Work out the finished part from the listing and answer in its coordinate system (mm). Coordinates: 2 decimals unless noted, no trailing zeros.
1. Find the intervals of material crossed by probe 1 along Y at (x, z) = (0.25, 0.2), in increasing order.
2. The part is cut by section A-A, the plane y = -2.75. Count the separate pieces of the cut face and the enclosed holes in it, then the cut area to 3 significant figures.
3. Determine the mould class of faces 1 (the flat face through (-14.286, -3.7, 0.5)), 2 (the flat face through (-17.111, -5.1, 0.5)), 3 (the flat face through (-2.686, -6.3, 0.5)) for opening direction X: +X half, -X half, draft (parallel to the pull), parting line (faces both ways), or undercut.
```python
from build123d import *

# Parameters (mm, degrees)
F1_W     = 20.491264
F1_H     = 6.716872
F1_W_2   = 0.4
F1_H_2   = 2.2
F2_DEPTH = 1


with BuildPart() as f2:
    # F1 (on face) → F2 (new body)
    with BuildSketch(Plane.XY):
        with Locations((-6.865435, -5.054062)):
            Rectangle(F1_W, F1_H)
        with Locations((-16.485979, -6.256568)):
            Rectangle(F1_W_2, F1_H_2, mode=Mode.SUBTRACT)
        with Locations((-15.685979, -6.256568)):
            Rectangle(F1_W_2, F1_H_2, mode=Mode.SUBTRACT)
        with Locations((-14.885979, -6.256568)):
            Rectangle(F1_W_2, F1_H_2, mode=Mode.SUBTRACT)
        with Locations((-14.085979, -6.256568)):
            Rectangle(F1_W_2, F1_H_2, mode=Mode.SUBTRACT)
        with Locations((-13.285979, -6.256568)):
            Rectangle(F1_W_2, F1_H_2, mode=Mode.SUBTRACT)
        with Locations((-12.485979, -6.256568)):
            Rectangle(F1_W_2, F1_H_2, mode=Mode.SUBTRACT)
        with Locations((-11.685979, -6.256568)):
            Rectangle(F1_W_2, F1_H_2, mode=Mode.SUBTRACT)
        with Locations((-10.885979, -6.256568)):
            Rectangle(F1_W_2, F1_H_2, mode=Mode.SUBTRACT)
        with Locations((-10.085979, -6.256568)):
            Rectangle(F1_W_2, F1_H_2, mode=Mode.SUBTRACT)
        with Locations((-9.285979, -6.256568)):
            Rectangle(F1_W_2, F1_H_2, mode=Mode.SUBTRACT)
        with Locations((-8.485979, -6.256568)):
            Rectangle(F1_W_2, F1_H_2, mode=Mode.SUBTRACT)
        with Locations((-7.685979, -6.256568)):
            Rectangle(F1_W_2, F1_H_2, mode=Mode.SUBTRACT)
        with Locations((-6.885979, -6.256568)):
            Rectangle(F1_W_2, F1_H_2, mode=Mode.SUBTRACT)
        with Locations((-16.485979, -3.656568)):
            Rectangle(F1_W_2, F1_H_2, mode=Mode.SUBTRACT)
        with Locations((-15.685979, -3.656568)):
            Rectangle(F1_W_2, F1_H_2, mode=Mode.SUBTRACT)
        with Locations((-14.885979, -3.656568)):
            Rectangle(F1_W_2, F1_H_2, mode=Mode.SUBTRACT)
        with Locations((-14.085979, -3.656568)):
            Rectangle(F1_W_2, F1_H_2, mode=Mode.SUBTRACT)
        with Locations((-13.285979, -3.656568)):
            Rectangle(F1_W_2, F1_H_2, mode=Mode.SUBTRACT)
        with Locations((-12.485979, -3.656568)):
            Rectangle(F1_W_2, F1_H_2, mode=Mode.SUBTRACT)
        with Locations((-11.685979, -3.656568)):
            Rectangle(F1_W_2, F1_H_2, mode=Mode.SUBTRACT)
        with Locations((-10.885979, -3.656568)):
            Rectangle(F1_W_2, F1_H_2, mode=Mode.SUBTRACT)
        with Locations((-10.085979, -3.656568)):
            Rectangle(F1_W_2, F1_H_2, mode=Mode.SUBTRACT)
        with Locations((-9.285979, -3.656568)):
            Rectangle(F1_W_2, F1_H_2, mode=Mode.SUBTRACT)
        with Locations((-8.485979, -3.656568)):
            Rectangle(F1_W_2, F1_H_2, mode=Mode.SUBTRACT)
        with Locations((-7.685979, -3.656568)):
            Rectangle(F1_W_2, F1_H_2, mode=Mode.SUBTRACT)
        with Locations((-6.885979, -3.656568)):
            Rectangle(F1_W_2, F1_H_2, mode=Mode.SUBTRACT)
        with Locations((-6.085979, -6.256568)):
            Rectangle(F1_W_2, F1_H_2, mode=Mode.SUBTRACT)
        with Locations((-5.285979, -6.256568)):
            Rectangle(F1_W_2, F1_H_2, mode=Mode.SUBTRACT)
        with Locations((-4.485979, -6.256568)):
            Rectangle(F1_W_2, F1_H_2, mode=Mode.SUBTRACT)
        with Locations((-3.685979, -6.256568)):
            Rectangle(F1_W_2, F1_H_2, mode=Mode.SUBTRACT)
        with Locations((-2.885979, -6.256568)):
            Rectangle(F1_W_2, F1_H_2, mode=Mode.SUBTRACT)
        with Locations((-2.085979, -6.256568)):
            Rectangle(F1_W_2, F1_H_2, mode=Mode.SUBTRACT)
        with Locations((-1.285979, -6.256568)):
            Rectangle(F1_W_2, F1_H_2, mode=Mode.SUBTRACT)
        with Locations((-0.485979, -6.256568)):
            Rectangle(F1_W_2, F1_H_2, mode=Mode.SUBTRACT)
        with Locations((0.314021, -6.256568)):
            Rectangle(F1_W_2, F1_H_2, mode=Mode.SUBTRACT)
        with Locations((1.114021, -6.256568)):
            Rectangle(F1_W_2, F1_H_2, mode=Mode.SUBTRACT)
        with Locations((1.914021, -6.256568)):
            Rectangle(F1_W_2, F1_H_2, mode=Mode.SUBTRACT)
        with Locations((2.714021, -6.256568)):
            Rectangle(F1_W_2, F1_H_2, mode=Mode.SUBTRACT)
        with Locations((-6.085979, -3.656568)):
            Rectangle(F1_W_2, F1_H_2, mode=Mode.SUBTRACT)
        with Locations((-5.285979, -3.656568)):
            Rectangle(F1_W_2, F1_H_2, mode=Mode.SUBTRACT)
        with Locations((-4.485979, -3.656568)):
            Rectangle(F1_W_2, F1_H_2, mode=Mode.SUBTRACT)
        with Locations((-3.685979, -3.656568)):
            Rectangle(F1_W_2, F1_H_2, mode=Mode.SUBTRACT)
        with Locations((-2.885979, -3.656568)):
            Rectangle(F1_W_2, F1_H_2, mode=Mode.SUBTRACT)
        with Locations((-2.085979, -3.656568)):
            Rectangle(F1_W_2, F1_H_2, mode=Mode.SUBTRACT)
        with Locations((-1.285979, -3.656568)):
            Rectangle(F1_W_2, F1_H_2, mode=Mode.SUBTRACT)
        with Locations((-0.485979, -3.656568)):
            Rectangle(F1_W_2, F1_H_2, mode=Mode.SUBTRACT)
        with Locations((0.314021, -3.656568)):
            Rectangle(F1_W_2, F1_H_2, mode=Mode.SUBTRACT)
        with Locations((1.114021, -3.656568)):
            Rectangle(F1_W_2, F1_H_2, mode=Mode.SUBTRACT)
        with Locations((1.914021, -3.656568)):
            Rectangle(F1_W_2, F1_H_2, mode=Mode.SUBTRACT)
        with Locations((2.714021, -3.656568)):
            Rectangle(F1_W_2, F1_H_2, mode=Mode.SUBTRACT)
    extrude(amount=F2_DEPTH)


solid = f2.part
```
Geometry says:
1. probe 1: y = -8.41 to -7.36, -5.16 to -4.76, -2.56 to -1.7
2. separate pieces: 26
2. enclosed holes: 0
2. area: 10.5 mm2
3. face 1: undercut
3. face 2: -X half
3. face 3: undercut
